Here's how the part is built. I have some questions about the finished solid (model axes, mm). Round coordinates to 2 decimals unless told otherwise and drop trailing zeros. Order: outer loops, then holes, each group sorted by start corner. A loop starts at its lowest first (then second) coordinate and runs counter-clockwise, first axis right, second up. Notation, with made-up numbers: (-11, -37.5) - (34, -37.5) arc R24 ccw to (34, -20.5) - close; hole circle Ø1 at (7.25, 8.25). An arc over 180 degrees is marked (long way). Answer as a JSON object with one key per item and string values.
```python
from build123d import *

# Parameters (mm, degrees)
SKETCH1_R           = 105
SKETCH1_R_2         = 53
SKETCH1_R_3         = 4
BOSS_EXTRUDE1_DEPTH = 4


with BuildPart() as part:
    # Sketch1 → Boss-Extrude1 (new body)
    with BuildSketch(Plane.XY):
        Circle(SKETCH1_R)
        Circle(SKETCH1_R_2, mode=Mode.SUBTRACT)
        with Locations((0, 58)):
            Circle(SKETCH1_R_3, mode=Mode.SUBTRACT)
        with Locations((30, 79.529868603)):
            Circle(SKETCH1_R_3, mode=Mode.SUBTRACT)
        with Locations((15, 93.808315196)):
            Circle(SKETCH1_R_3, mode=Mode.SUBTRACT)
        with Locations((58, 0)):
            Circle(SKETCH1_R_3, mode=Mode.SUBTRACT)
        with Locations((0, -58)):
            Circle(SKETCH1_R_3, mode=Mode.SUBTRACT)
        with Locations((-58, 0)):
            Circle(SKETCH1_R_3, mode=Mode.SUBTRACT)
        with Locations((77.449312832, 35.02290596)):
            Circle(SKETCH1_R_3, mode=Mode.SUBTRACT)
        with Locations((79.529868603, -30)):
            Circle(SKETCH1_R_3, mode=Mode.SUBTRACT)
        with Locations((35.02290596, -77.449312832)):
            Circle(SKETCH1_R_3, mode=Mode.SUBTRACT)
        with Locations((-30, -79.529868603)):
            Circle(SKETCH1_R_3, mode=Mode.SUBTRACT)
        with Locations((-77.449312832, -35.02290596)):
            Circle(SKETCH1_R_3, mode=Mode.SUBTRACT)
        with Locations((-79.529868603, 30)):
            Circle(SKETCH1_R_3, mode=Mode.SUBTRACT)
        with Locations((-35.02290596, 77.449312832)):
            Circle(SKETCH1_R_3, mode=Mode.SUBTRACT)
        with Locations((76.939097525, 55.725894089)):
            Circle(SKETCH1_R_3, mode=Mode.SUBTRACT)
        with Locations((93.808315196, -15)):
            Circle(SKETCH1_R_3, mode=Mode.SUBTRACT)
        with Locations((55.725894089, -76.939097525)):
            Circle(SKETCH1_R_3, mode=Mode.SUBTRACT)
        with Locations((-15, -93.808315196)):
            Circle(SKETCH1_R_3, mode=Mode.SUBTRACT)
        with Locations((-76.939097525, -55.725894089)):
            Circle(SKETCH1_R_3, mode=Mode.SUBTRACT)
        with Locations((-93.808315196, 15)):
            Circle(SKETCH1_R_3, mode=Mode.SUBTRACT)
        with Locations((-55.725894089, 76.939097525)):
            Circle(SKETCH1_R_3, mode=Mode.SUBTRACT)
    extrude(amount=BOSS_EXTRUDE1_DEPTH)


solid = part.part
```
1. Imagine slicing it at C-C (y = 86). List the corners of the cut face in (x, z) for me, plus the area to 3 significant figures.
Responses:
{"outline": "(-60.24, 0) - (60.24, 0) - (60.24, 4) - (-60.24, 4) - close", "area": "482 mm2"}
2. Imagine slicing it at A-A (y = -8.5). List the corners of the cut face in (x, z) for me, plus the area to 3 significant figures.
Responses:
{"outline": "(-104.66, 0) - (-52.31, 0) - (-52.31, 4) - (-104.66, 4) - close; (52.31, 0) - (104.66, 0) - (104.66, 4) - (52.31, 4) - close", "area": "419 mm2"}
3. If I drill on L1, parallel to Y at x = 0, z = 1.8; L2, parallel to X at y = 80, z = 0.75; L3, parallel to X at y = 76, z = 3.1, over which ranges is the centre line in solid material (lowest first)? Write a range as [from, to].
Responses:
{"L1": "[-105, -62], [-54, -53], [53, 54], [62, 105]", "L2": "[-68.01, -58.3], [-53.15, -38.1], [-31.94, 26.03], [33.97, 68.01]", "L3": "[-72.45, -59.61], [-51.84, -38.75], [-31.29, 28.12], [31.88, 72.45]"}
4. Imagine slicing it at B-B (x = -48). List the corners of the cut face in (y, z) for me.
Responses:
{"outline": "(-93.39, 0) - (-22.47, 0) - (-22.47, 4) - (-93.39, 4) - close; (22.47, 0) - (93.39, 0) - (93.39, 4) - (22.47, 4) - close"}
5. For P1, Ø1.5, axis at y = -63, z = 1, coming from the +X side, with a flat end and sliding along its axis, tell me the tip position at first contact or that it passes through.
Responses:
{"P1": "x = 84.56"}
6. Thinking about a two-plate mould opening in X: for faces 1 (the face through (100.15, 31.54, 1.97)), 2 (the face through (-48, 25, 4)), 3 (the face through (28, 45, 2)), which applies, pulls with the +X half, pulls with the -X half, needs draft (parallel to the pull), parting line crosses it, or undercut?
Responses:
{"face 1": "parting line crosses it", "face 2": "needs draft", "face 3": "undercut"}
